Source: CAD feature listing. Evaluate the final solid. Frame: model axes, mm. A direction names the side the tool comes from. Give positions to 0.01 mm unless a question says otherwise; leave off trailing zeros. Loops run counter-clockwise (first coordinate to the right, second up) from the corner with the lowest first, then second, coordinate; pieces in that order, holes last. Notation, with made-up numbers: (32.5, 35.5) -> (86.5, 35.5) arc R26 cw to (86.5, 65.5) -> close; hole circle Ø4 at (-36.5, 71.25). An arc over 180 degrees is marked (long way). Return JSON: item names as keys, results as strings. Group by question number.
(1) Cut plane B-B on x = -21. Return loops of the section in (y, z).
(2) Cut plane D-D on y = 26. Return loops of the section in (x, z), then the cut area to 3 significant figures.
(3) Pin query (flat end, axial travel): pin 1 (5 mm diameter, centred on y = 14.5, z = -2.5, fed in from +X); pin 2 (3 mm diameter, centred on y = -21, z = 1, fed in from +X); pin 3 (3 mm diameter, centred on y = 26.5, z = 1.5, fed in from -X). Return the tip coordinate at first contact, or that it passes through.
(4) Access query for faces 1 (the face through (0, -22, 0)), 2 (the face through (8, -8, -4.801)). Directions: +Z, -Z, +X, -X, +Y, -Y. A direction counts if a zero-diameter tool reaches every point of the face in a straight line with its end or side. Return the directions, or none.
(5) Draft query along X for faces 3 (the face through (-30.235, -23.183, 0.067)), 4 (the face through (-16, -16, 0)), 5 (the face through (8, -8, 4.801)). Return one class per face: released by +X, released by -X, zero draft, split by the parting line, or undercut.
(6) Ray query, line 1 (Y direction, x = -3, z = 0); line 2 (Y direction, x = -19.5, z = -2.5); line 3 (X direction, y = 17.5, z = -0.25). Return the intervals inside material, ascending. Write a range as from..to.
(7) Cut plane C-C on y = -16.5. Return loops of the section in (x, z).
(8) Cut plane A-A on z = 2.25. Return loops of the section in (x, y).
```python
from build123d import *

# Parameters (mm, degrees)
F0_R     = 38.1
F1_DEPTH = 4.8006
F3_R     = 11.049
F4_DEPTH = 25.4
F5_DEPTH = 25.4


with BuildPart() as f1:
    # F0 (on Top) → F1 (new body, symmetric)
    with BuildSketch(Plane.XY):
        Circle(F0_R)
    extrude(amount=F1_DEPTH, both=True)

    # F3 (on face) → F4 (cut)
    with BuildSketch(Plane.XY.offset(4.8006)):
        Circle(F3_R)
    extrude(amount=-F4_DEPTH, mode=Mode.SUBTRACT)

    # F2 (on face) → F5 (cut)
    with BuildSketch(Plane.XY.offset(4.8006)):
        with BuildLine():
            ThreePointArc((17.9605122421, 17.9605122421), (23.4665401258, 9.7201591821), (25.4, 0))
            Line((25.4, 0), (31.75, 0))
            ThreePointArc((31.75, 0), (29.3331751572, 12.1501989776), (22.4506403027, 22.4506403027))
            Line((22.4506403027, 22.4506403027), (17.9605122421, 17.9605122421))
        make_face()
        with BuildLine():
            ThreePointArc((-17.9605122421, 17.9605122421), (-9.7201591821, 23.4665401258), (0, 25.4))
            Line((0, 25.4), (0, 31.75))
            ThreePointArc((0, 31.75), (-12.1501989776, 29.3331751572), (-22.4506403027, 22.4506403027))
            Line((-22.4506403027, 22.4506403027), (-17.9605122421, 17.9605122421))
        make_face()
        with BuildLine():
            Line((-22.4506403027, -22.4506403027), (-17.9605122421, -17.9605122421))
            ThreePointArc((-17.9605122421, -17.9605122421), (-23.4665401258, -9.7201591821), (-25.4, 0))
            Line((-25.4, 0), (-31.75, 0))
            ThreePointArc((-31.75, 0), (-29.3331751572, -12.1501989776), (-22.4506403027, -22.4506403027))
        make_face()
        with BuildLine():
            Line((22.4506403027, -22.4506403027), (17.9605122421, -17.9605122421))
            ThreePointArc((17.9605122421, -17.9605122421), (9.7201591821, -23.4665401258), (0, -25.4))
            Line((0, -25.4), (0, -31.75))
            ThreePointArc((0, -31.75), (12.1501989776, -29.3331751572), (22.4506403027, -22.4506403027))
        make_face()
        with BuildLine():
            Line((-13.4703841816, -13.4703841816), (-8.9802561211, -8.9802561211))
            ThreePointArc((-8.9802561211, -8.9802561211), (-11.7332700629, -4.860079591), (-12.7, 0))
            Line((-12.7, 0), (-19.05, 0))
            ThreePointArc((-19.05, 0), (-17.5999050943, -7.2901193866), (-13.4703841816, -13.4703841816))
        make_face()
        with BuildLine():
            ThreePointArc((-8.9802561211, 8.9802561211), (-4.860079591, 11.7332700629), (0, 12.7))
            Line((0, 12.7), (0, 19.05))
            ThreePointArc((0, 19.05), (-7.2901193866, 17.5999050943), (-13.4703841816, 13.4703841816))
            Line((-13.4703841816, 13.4703841816), (-8.9802561211, 8.9802561211))
        make_face()
        with BuildLine():
            ThreePointArc((8.9802561211, 8.9802561211), (11.7332700629, 4.860079591), (12.7, 0))
            Line((12.7, 0), (19.05, 0))
            ThreePointArc((19.05, 0), (17.5999050943, 7.2901193866), (13.4703841816, 13.4703841816))
            Line((13.4703841816, 13.4703841816), (8.9802561211, 8.9802561211))
        make_face()
        with BuildLine():
            Line((13.4703841816, -13.4703841816), (8.9802561211, -8.9802561211))
            ThreePointArc((8.9802561211, -8.9802561211), (4.860079591, -11.7332700629), (0, -12.7))
            Line((0, -12.7), (0, -19.05))
            ThreePointArc((0, -19.05), (7.2901193866, -17.5999050943), (13.4703841816, -13.4703841816))
        make_face()
        with BuildLine():
            ThreePointArc((-13.4703841816, 13.4703841816), (-7.2901193866, 17.5999050943), (0, 19.05))
            Line((0, 19.05), (0, 25.4))
            ThreePointArc((0, 25.4), (-9.7201591821, 23.4665401258), (-17.9605122421, 17.9605122421))
            Line((-17.9605122421, 17.9605122421), (-13.4703841816, 13.4703841816))
        make_face()
        with BuildLine():
            ThreePointArc((13.4703841816, 13.4703841816), (17.5999050943, 7.2901193866), (19.05, 0))
            Line((19.05, 0), (25.4, 0))
            ThreePointArc((25.4, 0), (23.4665401258, 9.7201591821), (17.9605122421, 17.9605122421))
            Line((17.9605122421, 17.9605122421), (13.4703841816, 13.4703841816))
        make_face()
        with BuildLine():
            Line((-17.9605122421, -17.9605122421), (-13.4703841816, -13.4703841816))
            ThreePointArc((-13.4703841816, -13.4703841816), (-17.5999050943, -7.2901193866), (-19.05, 0))
            Line((-19.05, 0), (-25.4, 0))
            ThreePointArc((-25.4, 0), (-23.4665401258, -9.7201591821), (-17.9605122421, -17.9605122421))
        make_face()
        with BuildLine():
            Line((17.9605122421, -17.9605122421), (13.4703841816, -13.4703841816))
            ThreePointArc((13.4703841816, -13.4703841816), (7.2901193866, -17.5999050943), (0, -19.05))
            Line((0, -19.05), (0, -25.4))
            ThreePointArc((0, -25.4), (9.7201591821, -23.4665401258), (17.9605122421, -17.9605122421))
        make_face()
    extrude(amount=-F5_DEPTH, mode=Mode.SUBTRACT)


solid = f1.part
```
Answers:
{
 "1": {"outline": "(-31.79, -4.8) -> (-21, -4.8) -> (-21, 4.8) -> (-31.79, 4.8) -> close; (0, -4.8) -> (21, -4.8) -> (21, 4.8) -> (0, 4.8) -> close; (23.81, -4.8) -> (31.79, -4.8) -> (31.79, 4.8) -> (23.81, 4.8) -> close"},
 "2": {"outline": "(-27.85, -4.8) -> (-18.22, -4.8) -> (-18.22, 4.8) -> (-27.85, 4.8) -> close; (0, -4.8) -> (27.85, -4.8) -> (27.85, 4.8) -> (0, 4.8) -> close", "area": "360 mm²"},
 "3": {"pin 1": "x = 36.16", "pin 2": "x = 32.73", "pin 3": "x = -28.75"},
 "4": {"face 1": "+Z, -Z", "face 2": "-Z, +X, -X, +Y, -Y"},
 "5": {"face 3": "split by the parting line", "face 4": "undercut", "face 5": "zero draft"},
 "6": {"line 1": "-37.98..-10.63, 10.63..12.34, 31.61..37.98", "line 2": "-32.73..-19.5, 0..19.5, 25.06..32.73", "line 3": "-33.84..-17.5, 0..17.5, 26.49..33.84"},
 "7": {"outline": "(-34.34, -4.8) -> (-27.13, -4.8) -> (-27.13, 4.8) -> (-34.34, 4.8) -> close; (-16.5, -4.8) -> (0, -4.8) -> (0, 4.8) -> (-16.5, 4.8) -> close; (16.5, -4.8) -> (34.34, -4.8) -> (34.34, 4.8) -> (16.5, 4.8) -> close"},
 "8": {"outline": "circle Ø76.2 at (0, 0); hole (-31.75, 0) arc R31.75 ccw to (-22.45, -22.45) -> (-8.98, -8.98) arc R12.7 cw to (-12.7, 0) -> close; hole (-22.45, 22.45) -> (-8.98, 8.98) arc R12.7 cw to (0, 12.7) -> (0, 31.75) arc R31.75 ccw to start; hole circle Ø22.1 at (0, 0); hole (0, -31.75) arc R31.75 ccw to (22.45, -22.45) -> (8.98, -8.98) arc R12.7 cw to (0, -12.7) -> close; hole (8.98, 8.98) arc R12.7 cw to (12.7, 0) -> (31.75, 0) arc R31.75 ccw to (22.45, 22.45) -> close"}
}
